Geometry check sheet. Reference: the model listing, model coordinates, mm. Round coordinates to 2 decimals unless told otherwise and drop trailing zeros. Order: outer loops, then holes, each group sorted by start corner. A loop starts at its lowest first (then second) coordinate and runs counter-clockwise, first axis right, second up. Notation, with made-up numbers: (75.25, 39) - (94.25, 39) arc R34 ccw to (94.25, 71) - close; hole circle Ø2 at (-6, 36). An arc over 180 degrees is marked (long way). One line per question, with ' | ' between items. Start each with the question number.
Q1. Sectioned sample at C-C, the plane x = 66. Enter the section's corners in (y, z), then the cut area to 3 significant figures.
Q2. Sectioned sample at D-D, the plane z = 131. Enter the section's corners in (x, y).
Q3. Gauge pin test, flat ends, axial feed: P1, Ø3, axis at x = 82.5, z = 44, coming from the +Y side; P2, Ø2.5, axis at x = 47.5, y = -1.5, coming from the +Z side. Record the tip position at first contact, or that the pin passes through.
Q4. Sectioned sample at A-A, the plane z = -44.45. Enter the section's corners in (x, y).
Q5. Material ranges on line 1 along X through (y, z) = (-1.5, -25.5); line 2 along Z through (x, y) = (-79.5, -0.6); line 3 along Z through (x, y) = (-101, -0.95), recorded low to high.
```python
from build123d import *

# Parameters (mm, degrees)
F1_DEPTH = 4.7625


with BuildPart() as f1:
    # F0 (on Front) → F1 (new body)
    with BuildSketch(Plane.XZ):
        with BuildLine():
            Line((-66.415057, 228.6), (-117.215057, 228.6))
            Line((-117.215057, 228.6), (-117.215057, 150.698523))
            ThreePointArc((-117.215057, 150.698523), (-104.037951, 150.408904), (-98.21409, 138.585087))
            Line((-98.21409, 138.585087), (-98.21409, 102.387595))
            ThreePointArc((-98.21409, 102.387595), (-101.38909, 99.212595), (-104.564089, 102.387595))
            Line((-104.564089, 102.387595), (-104.564089, 138.912405))
            Line((-104.564089, 138.912405), (-104.564089, 140.487595))
            ThreePointArc((-104.564089, 140.487595), (-111.259617, 146.03773), (-117.215057, 139.7))
            Line((-117.215057, 139.7), (-117.215057, 23.698523))
            ThreePointArc((-117.215057, 23.698523), (-104.345751, 23.599021), (-98.17113, 12.307299))
            Line((-98.17113, 12.307299), (-98.17113, -25.122353))
            ThreePointArc((-98.17113, -25.122353), (-101.34613, -28.297353), (-104.52113, -25.122353))
            Line((-104.52113, -25.122353), (-104.52113, 12.422353))
            Line((-104.52113, 12.422353), (-104.52113, 12.977647))
            ThreePointArc((-104.52113, 12.977647), (-111.003914, 19.048482), (-117.215057, 12.7))
            Line((-117.215057, 12.7), (-117.215057, -50.8))
            Line((-117.215057, -50.8), (-53.715057, -50.8))
            ThreePointArc((-53.715057, -50.8), (-47.370554, -44.185833), (-54.242934, -38.121979))
            Line((-54.242934, -38.121979), (-92.342934, -38.121979))
            ThreePointArc((-92.342934, -38.121979), (-95.517934, -34.946979), (-92.342934, -31.771979))
            Line((-92.342934, -31.771979), (-54.461912, -31.771979))
            ThreePointArc((-54.461912, -31.771979), (-42.908089, -37.77921), (-42.716534, -50.8))
            Line((-42.716534, -50.8), (73.284943, -50.8))
            ThreePointArc((73.284943, -50.8), (79.611961, -43.910237), (72.209324, -38.191762))
            Line((72.209324, -38.191762), (34.109324, -38.191762))
            ThreePointArc((34.109324, -38.191762), (30.934324, -35.016762), (34.109324, -31.841762))
            Line((34.109324, -31.841762), (71.761023, -31.841762))
            ThreePointArc((71.761023, -31.841762), (83.881911, -37.450409), (84.283466, -50.8))
            Line((84.283466, -50.8), (162.184943, -50.8))
            Line((162.184943, -50.8), (162.184943, 0))
            Line((162.184943, 0), (149.484943, 12.7))
            Line((149.484943, 12.7), (149.484943, -25.502864))
            ThreePointArc((149.484943, -25.502864), (146.309943, -28.677864), (143.134943, -25.502864))
            Line((143.134943, -25.502864), (143.134943, 19.05))
            Line((143.134943, 19.05), (-66.415057, 228.6))
        make_face()
    extrude(amount=F1_DEPTH)


solid = f1.part
```
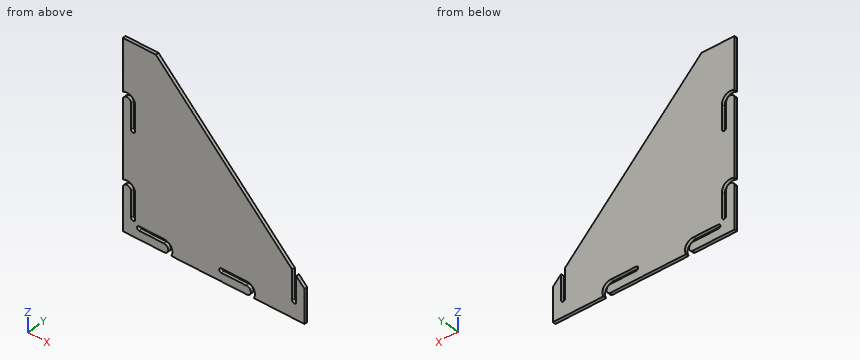
Determined:
1) outline: (-4.76, -50.8) - (0, -50.8) - (0, -38.19) - (-4.76, -38.19) - close; (-4.76, -31.84) - (0, -31.84) - (0, 96.18) - (-4.76, 96.18) - close | area: 670 mm2
2) outline: (-117.22, -4.76) - (-104.56, -4.76) - (-104.56, 0) - (-117.22, 0) - close; (-98.21, -4.76) - (31.18, -4.76) - (31.18, 0) - (-98.21, 0) - close
3) P1: stops at y = 0 | P2: stops at z = 115.93
4) outline: (-117.22, -4.76) - (-47.37, -4.76) - (-47.37, 0) - (-117.22, 0) - close; (-41.02, -4.76) - (79.63, -4.76) - (79.63, 0) - (-41.02, 0) - close; (85.98, -4.76) - (162.18, -4.76) - (162.18, 0) - (85.98, 0) - close
5) line 1: x = -117.22 to -104.5, -98.19 to 143.13, 149.48 to 162.18 | line 2: z = -50.8 to -38.12, -31.77 to 228.6 | line 3: z = -50.8 to -28.28, 20.7 to 99.24, 147.7 to 228.6
